The listing builds one solid part. Answer for the finished solid, in the listing's coordinates (mm). Give positions to 0.01 mm unless a question says otherwise; leave off trailing zeros. Order: outer loops, then holes, each group sorted by start corner. A loop starts at its lowest first (then second) coordinate and runs counter-clockwise, first axis right, second up. Notation, with made-up numbers: (2, 12) - (46, 12) arc R6 cw to (46, 23) - close; hole circle Ø8 at (45, 44). An arc over 180 degrees is marked (long way). Write each question's results on one line, items separated by ' | '. Start each with the question number.
1. Section D-D (x = -31.45) is taken. Give the vertices of the cut face in (y, z), and give its area (3 significant figures).
2. Section C-C (z = 1.45) is taken. Give the vertices of the cut face in (x, y), and give its area (3 significant figures).
3. Section B-B (x = -29) is taken. Give the vertices of the cut face in (y, z).
4. Determine the mould class of faces 1 (the face through (-27.467, 3.178, 2.504)), 2 (the face through (-31, 5, 0)), 3 (the face through (-31.082, 4.207, 2.576)) for opening direction X: released by +X, released by -X, zero draft, split by the parting line, or undercut.
5. Flat-ended cylindrical pins translate along their axes: pin 1 (2 mm diameter, centred on x = -28.5, z = 3, fed in from -Y); pin 2 (1.5 mm diameter, centred on x = -31.5, z = 1.5, fed in from +Y); pin 3 (3 mm diameter, centred on x = -28, y = 3, fed in from -Z). Find the tip coordinate at first contact, or state that the pin passes through.
6. Section A-A (y = 3.5) is taken. Give the vertices of the cut face in (x, z).
7. Find the intervals of material crossed by L1, parallel to X at y = 3.25, z = 0.2; L2, parallel to Y at x = -30.2, z = 2.8; L3, parallel to X at y = 3.95, z = 0.8, in increasing order.
from build123d import *

# Parameters (mm, degrees)
F0_R     = 12.192
F1_DEPTH = 24.13
F3_R     = 2.54
F4_DEPTH = 5.08
F5_R     = 1.27
F6_DEPTH = 12.7


with BuildPart() as f1:
    # F0 (on Top) → F1 (new body)
    with BuildSketch(Plane.XY):
        with Locations((-42.4534301028, 33.8528162107)):
            Circle(F0_R)
    extrude(amount=F1_DEPTH)


with BuildPart() as f4:
    # F3 (on Top) → F4 (new body)
    with BuildSketch(Plane.XY):
        with Locations((-29.813402482, 4.1510883982)):
            Circle(F3_R)
    extrude(amount=F4_DEPTH)

    # F5 (on Top) → F6 (cut, symmetric)
    with BuildSketch(Plane.XY):
        with Locations((-29.813402482, 4.1510883982)):
            Circle(F5_R)
    extrude(amount=F6_DEPTH, both=True, mode=Mode.SUBTRACT)


solid = f4.part
Reported:
1) outline: (2.21, 0) - (6.09, 0) - (6.09, 5.08) - (2.21, 5.08) - close | area: 19.7 mm²
2) outline: circle Ø5.08 at (-29.81, 4.15); hole circle Ø2.54 at (-29.81, 4.15) | area: 15.2 mm²
3) outline: (1.74, 0) - (3.18, 0) - (3.18, 5.08) - (1.74, 5.08) - close; (5.13, 0) - (6.56, 0) - (6.56, 5.08) - (5.13, 5.08) - close
4) face 1: split by the parting line | face 2: zero draft | face 3: undercut
5) pin 1: y = 1.63 | pin 2: y = 6.51 | pin 3: z = 0
6) outline: (-32.27, 0) - (-30.9, 0) - (-30.9, 5.08) - (-32.27, 5.08) - close; (-28.72, 0) - (-27.36, 0) - (-27.36, 5.08) - (-28.72, 5.08) - close
7) L1: -32.19 to -30.71, -28.92 to -27.44 | L2: 1.64 to 2.94, 5.36 to 6.66 | L3: -32.35 to -31.07, -28.56 to -27.28
